```python
from build123d import *

# Parameters (mm, degrees)
PAD_DEPTH       = 25
CHAMFER_SIZE    = 5
PAD001_DEPTH    = 2.5
SKETCH002_R     = 11
POCKET_DEPTH    = 5
SKETCH003_R     = 1.75
HOLE_DEPTH      = 25
POCKET001_DEPTH = 5


with BuildPart() as part:
    # Sketch → Pad (new body, symmetric)
    with BuildSketch(Plane.YZ):
        Polygon((0, 51), (0, 0), (-54, 0), (-54, 2.75), (-2.75, 2.75), (-2.75, 51), align=None)
    extrude(amount=PAD_DEPTH, both=True)

    # Chamfer
    chamfer_edges = [part.edges().sort_by_distance(p)[0] for p in [
        (25, -1.375, 51),
        (-25, -1.375, 51),
        (25, -54, 1.375),
        (-25, -54, 1.375),
    ]]
    chamfer(chamfer_edges, length=CHAMFER_SIZE)

    # Sketch001 (on Face6 of Chamfer) → Pad001 (join)
    with BuildSketch(Plane.YZ.offset(25)):
        Polygon((-2.75, 2.75), (-2.75, 22.75), (-17.75, 2.75), align=None)
    pad001 = extrude(amount=-PAD001_DEPTH)

    # Mirrored: Pad001 across YZ
    add(pad001.mirror(Plane.YZ))

    # Sketch002 (on Face7 of Mirrored) → Pocket (cut)
    with BuildSketch(Plane(origin=(0, -2.75, 0), x_dir=(0, 0, -1), z_dir=(0, -1, 0))):
        with Locations((-29.8, 0)):
            Circle(SKETCH002_R)
    extrude(amount=-POCKET_DEPTH, mode=Mode.SUBTRACT)

    # Sketch003 (on Face9 of Pocket) → Hole (cut)
    with BuildSketch(Plane(origin=(0, -2.75, 0), x_dir=(0, 0, -1), z_dir=(0, -1, 0))):
        with Locations((-45.3, 15.5)):
            Circle(SKETCH003_R)
        with Locations((-14.3, 15.5)):
            Circle(SKETCH003_R)
        with Locations((-14.3, -15.5)):
            Circle(SKETCH003_R)
        with Locations((-45.3, -15.5)):
            Circle(SKETCH003_R)
    extrude(amount=-HOLE_DEPTH, mode=Mode.SUBTRACT)

    # Sketch004 (on Face15 of Hole) → Pocket001 (cut)
    with BuildSketch(Plane(origin=(0, 0, 2.75), x_dir=(0, -1, 0), z_dir=(0, 0, 1))):
        with BuildLine():
            ThreePointArc((14, 17.25), (11.6, 14.85), (14, 12.45))
            Line((14, 12.45), (44, 12.45))
            ThreePointArc((44, 12.45), (46.4, 14.85), (44, 17.25))
            Line((14, 17.25), (44, 17.25))
        make_face()
        with BuildLine():
            ThreePointArc((14, -12.45), (11.6, -14.85), (14, -17.25))
            Line((14, -17.25), (44, -17.25))
            ThreePointArc((44, -17.25), (46.4, -14.85), (44, -12.45))
            Line((14, -12.45), (44, -12.45))
        make_face()
    extrude(amount=-POCKET001_DEPTH, mode=Mode.SUBTRACT)


solid = part.part
```
Source: CAD feature listing. Evaluate the final solid. Frame: model axes, mm. A direction names the side the tool comes from. Round coordinates to 2 decimals unless told otherwise and drop trailing zeros. Write each loop counter-clockwise with the first axis right and the second up, starting at its lowest first coordinate (ties: lowest second). Pieces come first, ordered by that corner, then holes. Notation, with made-up numbers: M 31,21 L 41,21 A4 ccw 41,25 Z; hole C 13.5,50 d2. An arc over 180 degrees is marked long. Answer as a JSON object with one key per item and string values. Group by question number.
(1) Mould query, pull axis Z, two halves, no side actions, for faces 4 (the flat face through (23.768, -10.145, 12.89)), 5 (the flat face through (0, -27, 0)), 6 (the flat face through (0, -54, 1)), 7 (the cylindrical face through (-13.765, -1.394, 14.528)). Classes: +Z half, -Z half, draft (parallel to the pull), parting line (faces both ways), or undercut.
(2) Section query C-C on x = 0. Output: boundary loops of the cut face in (y, z).
(3) Section query B-B on y = -41.5. Output: boundary loops of the cut face in (x, z).
(4) Section query D-D on x = -15.5. Output: boundary loops of the cut face in (y, z), then the cut area to 3 significant figures.
(5) Reachability of faces 1 (the flat face through (22, -52, 1)), 2 (the flat face through (-11, -2.75, 27)), 3 (the cylindrical face through (-14.9, -46.4, 1.4)) from +Z, -Z, +X, -X, +Y, -Y: full face, straight path, thin tool, end or side. Return the list, or none.
(6) Ray query, line 1 (X direction, y = -1.7, z = 45.3); line 2 (Z direction, x = -15, y = -1); line 3 (Z direction, x = 9.5, y = -31.5). Return the intervals inside material, ascending. Write a range as [from, to].
(7) Section query A-A on z = 29.8. Output: boundary loops of the cut face in (x, y), then the cut area to 3 significant figures.
(8) First-contact query: pin 1 (2 mm diameter, centred on x = 14, z = 32.5, fed in from -Y); pin 2 (6 mm diameter, centred on x = 17, y = -40.5, fed in from +Z). Flat tips, straight axial feed; report the tip coordinate or a pass-through.
Computed values:
{
 "1": {"face 4": "+Z half", "face 5": "-Z half", "face 6": "draft", "face 7": "undercut"},
 "2": {"outline": "M -54,0 L 0,0 L 0,18.8 L -2.75,18.8 L -2.75,2.75 L -54,2.75 Z; M -2.75,40.8 L 0,40.8 L 0,51 L -2.75,51 Z"},
 "3": {"outline": "M -25,0 L -17.25,0 L -17.25,2.75 L -25,2.75 Z; M -12.45,0 L 12.45,0 L 12.45,2.75 L -12.45,2.75 Z; M 17.25,0 L 25,0 L 25,2.75 L 17.25,2.75 Z"},
 "4": {"outline": "M -54,0 L -46.31,0 L -46.31,2.75 L -54,2.75 Z; M -11.69,0 L 0,0 L 0,12.55 L -2.75,12.55 L -2.75,2.75 L -11.69,2.75 Z; M -2.75,16.05 L 0,16.05 L 0,43.55 L -2.75,43.55 Z; M -2.75,47.05 L 0,47.05 L 0,51 L -2.75,51 Z", "area": "167 mm^2"},
 "5": {"face 1": "+Z, -Z, +X, -Y", "face 2": "+Z, -Y", "face 3": "+Z, -Z"},
 "6": {"line 1": "[-25, -17.25], [-13.75, 13.75], [17.25, 25]", "line 2": "[0, 12.62], [15.98, 43.62], [46.98, 51]", "line 3": "[0, 2.75]"},
 "7": {"outline": "M -25,-2.75 L -11,-2.75 L -11,0 L -25,0 Z; M 11,-2.75 L 25,-2.75 L 25,0 L 11,0 Z", "area": "77.0 mm^2"},
 "8": {"pin 1": "y = -2.75", "pin 2": "z = 2.75"}
}
